from build123d import *

# Parameters (mm, degrees)
BOSS_EXTRUDE1_DEPTH = 25
SKETCH2_R           = 1.5
CUT_EXTRUDE1_DEPTH  = 19
SKETCH3_R           = 1.5
BOSS_EXTRUDE2_DEPTH = 6


with BuildPart() as part:
    # Sketch1 → Boss-Extrude1 (new body)
    with BuildSketch(Plane(origin=(0, 0, 0), x_dir=(1, 0, 0), z_dir=(0, 1, 0))):
        Polygon((0, -2.309401077), (2, -1.154700538), (2, 1.154700538), (0, 2.309401077), (-2, 1.154700538), (-2, -1.154700538), align=None)
    extrude(amount=BOSS_EXTRUDE1_DEPTH)

    # Sketch2 → Cut-Extrude1 (cut)
    with BuildSketch(Plane(origin=(0, 25, 0), x_dir=(1, 0, 0), z_dir=(0, 1, 0))):
        Circle(SKETCH2_R)
    extrude(amount=-CUT_EXTRUDE1_DEPTH, mode=Mode.SUBTRACT)

    # Sketch3 → Boss-Extrude2 (add)
    with BuildSketch(Plane.XZ):
        Circle(SKETCH3_R)
    extrude(amount=BOSS_EXTRUDE2_DEPTH)


solid = part.part
Build history of the part. All positions in model axes, mm. A direction names the side the tool comes from. Give positions to 0.01 mm unless a question says otherwise; leave off trailing zeros. Loops run counter-clockwise (first coordinate to the right, second up) from the corner with the lowest first, then second, coordinate; pieces in that order, holes last. Notation, with made-up numbers: (-17, -5) - (35, -5) arc R19 cw to (35, 29) - close; hole circle Ø1 at (32.25, 56.25). An arc over 180 degrees is marked (long way). Write item = value, one per line. Start each with the question number.
1) Band-saw the part on C-C on x = -1.2. Give the cut face in (y, z), plus the area to 3 significant figures.
2) Tool access for faces 1 (the flat face through (-2, 12, 0)), 2 (the flat face through (0, 0, 2)), 3 (the flat face through (0, 6, 0)): list every direction of +Z, -Z, +X, -X, +Y, -Y with a clear straight run to the whole face (end or side of a thin tool).
3) Band-saw the part on D-D on y = 2.5. Give the cut face in (x, z), plus the area to 3 significant figures.
4) Pull direction X, two halves, no side cores. Call faces 4 (the cylindrical face through (-1.5, -2.96, 0.07)), 5 (the flat face through (0, 25, 2)), 6 (the cylindrical face through (-1.5, 15.63, -0.07)): +X half, -X half, draft (parallel to the pull), parting line (faces both ways), or undercut.
5) Band-saw the part on B-B on z = -0.9. Give the cut face in (x, y).
6) Drop flat-ended pins along their axis: pin 1 Ø1 at (x, y) = (-1.5, 9) entering from -Z; pin 2 Ø2 at (x, y) = (-0.5, 4.5) entering from -Z. Give the stop position or say it passes through.
7) Band-saw the part on A-A on y = 13.5. Give the cut face in (x, z), plus the area to 3 significant figures.
8) Probe probe 1 along X at (y, z) = (10.75, 0); probe 2 along X at (y, z) = (15, 0.6); probe 3 along Y at (x, z) = (0.7, -1.05). List the from-to ranges inside material, lowest first. Write a range as from..to.
Final values:
q1.outline = (-6, -0.9) - (0, -0.9) - (0, -1.62) - (25, -1.62) - (25, -0.9) - (6, -0.9) - (6, 0.9) - (25, 0.9) - (25, 1.62) - (0, 1.62) - (0, 0.9) - (-6, 0.9) - close
q1.area = 57.4 mm²
q2.face_1 = +Z, -Z, -X, +Y, -Y
q2.face_2 = -Y
q2.face_3 = +Y
q3.outline = (-2, -1.15) - (0, -2.31) - (2, -1.15) - (2, 1.15) - (0, 2.31) - (-2, 1.15) - close
q3.area = 13.9 mm²
q4.face_4 = parting line
q4.face_5 = draft
q4.face_6 = undercut
q5.outline = (-2, 0) - (-1.2, 0) - (-1.2, -6) - (1.2, -6) - (1.2, 0) - (2, 0) - (2, 25) - (1.2, 25) - (1.2, 6) - (-1.2, 6) - (-1.2, 25) - (-2, 25) - close
q6.pin_1 = -1.73
q6.pin_2 = -2.31
q7.outline = (-2, -1.15) - (0, -2.31) - (2, -1.15) - (2, 1.15) - (0, 2.31) - (-2, 1.15) - close; hole circle Ø3 at (0, 0)
q7.area = 6.79 mm²
q8.probe_1 = -2..-1.5, 1.5..2
q8.probe_2 = -2..-1.37, 1.37..2
q8.probe_3 = -6..6
